from build123d import *

# Parameters (mm, degrees)
SKETCH1_R           = 3.5
BASEHEAD_DEPTH      = 4
SKETCH2_R           = 2
BASEBODY_DEPTH      = 35
HEXAGONSOCKET_DEPTH = 2
TOPFILLET_R         = 0.5
CHAMFER1_SIZE       = 0.2
LPATTERN10_COUNT    = 44
LPATTERN10_PITCH    = 0.4548


with BuildPart() as part:
    # Sketch1 → BaseHead (new body)
    with BuildSketch(Plane(origin=(0, 0, 0), x_dir=(0, 0, -1), z_dir=(1, 0, 0))):
        Circle(SKETCH1_R)
    extrude(amount=BASEHEAD_DEPTH)

    # Sketch2 → BaseBody (add)
    with BuildSketch(Plane(origin=(4, 0, 0), x_dir=(0, 0, -1), z_dir=(1, 0, 0))):
        Circle(SKETCH2_R)
    extrude(amount=BASEBODY_DEPTH)

    # Sketch3 → HexagonSocket (cut)
    with BuildSketch(Plane(origin=(0, 0, 0), x_dir=(0, 0, -1), z_dir=(1, 0, 0))):
        Polygon((1.732050808, 0), (0.866025404, 1.5), (-0.866025404, 1.5), (-1.732050808, 0), (-0.866025404, -1.5), (0.866025404, -1.5), align=None)
    extrude(amount=HEXAGONSOCKET_DEPTH, mode=Mode.SUBTRACT)

    # Sketch4 → Cut-Revolve1 (revolve, cut)
    with BuildSketch(Plane(origin=(-4.19613823, 0.75, 0), x_dir=(-1, 0, 0), z_dir=(0, 0, 1)), mode=Mode.PRIVATE) as cut_revolve1_sk:
        Polygon((-6.19613823, 2.25), (-7.062163633, 0.75), (-6.19613823, 0.75), align=None)
    revolve(cut_revolve1_sk.sketch.rotate(Axis((0.838992387, 0, 0), (-1, 0, 0)), 90), axis=Axis((0.838992387, 0, 0), (-1, 0, 0)), mode=Mode.SUBTRACT)

    # TopFillet
    topfillet_edges = [part.edges().sort_by_distance(p)[0] for p in [
        (0, 0, 3.5),
    ]]
    fillet(topfillet_edges, radius=TOPFILLET_R)

    # Chamfer1
    chamfer1_edges = [part.edges().sort_by_distance(p)[0] for p in [
        (39, 0, 2),
    ]]
    chamfer(chamfer1_edges, length=CHAMFER1_SIZE)

    # Sketch5 → Cut-Revolve10 (revolve, cut)
    with BuildSketch(Plane.XY, mode=Mode.PRIVATE) as cut_revolve10_sk:
        Polygon((38.8, 1.671776372), (38.9895, 2), (38.9895, 2.379), (38.6105, 2.379), (38.6105, 2), align=None)
    cut_revolve10 = revolve(cut_revolve10_sk.sketch.rotate(Axis((0, 0, 0), (1, 0, 0)), 90), axis=Axis((0, 0, 0), (1, 0, 0)), mode=Mode.SUBTRACT)

    # LPattern10: Cut-Revolve10 ×44
    with Locations(*[(-i * LPATTERN10_PITCH, 0, 0) for i in range(1, LPATTERN10_COUNT)]):
        add(cut_revolve10, mode=Mode.SUBTRACT)


solid = part.part
Design review of the part built by this model. Coordinates are the model's own, in mm. Give positions to 0.01 mm unless a question says otherwise; leave off trailing zeros. Loops run counter-clockwise (first coordinate to the right, second up) from the corner with the lowest first, then second, coordinate; pieces in that order, holes last. Notation, with made-up numbers: (-12, 0.25) - (19, 0.25) arc R11 cw to (19, 8.25) - close; hole circle Ø3 at (71, 28). An arc over 180 degrees is marked (long way). Use CSV: the item, a comma, the result in double quotes. Start each with the question number.
1. Draft analysis for pull direction Y (two halves, no side actions). For faces 1 (the flat face through (0.986, -0.74, 1.305)), 2 (the flat face through (0, -1.3, -1.3)), state which applies: released by +Y, released by -Y, zero draft, split by the parting line, or undercut.
2. Add section A-A (x = 14). State the section outline as (y, z) points, plus the area to 3 significant figures.
3. Insertion check: P1, Ø1.5, axis at x = 7.5, z = 1.5, coming from the +Y side; P2, Ø0.6, axis at y = 1, z = -1, coming from the -X side; P3, Ø0.6, axis at y = -1, z = -0.5, coming from the -X side; P4, Ø3, axis at x = 10.5, z = 0, coming from the -Y side. Each pin has a flat end and moves straight along its axis. Give the tip position at first contact, or say it passes through.
4. Wall thickness on L1, parallel to X at y = 2.75, z = -0.5; L2, parallel to Y at x = 21, z = 0; L3, parallel to Z at x = 3.5, y = -1.75: over which ranges is each line inside the solid? List them lowest first.
Results found:
1,face 1,"undercut"
1,face 2,"zero draft"
2,outline,"circle Ø4 at (0, 0)"
2,area,"12.6 mm²"
3,P1,"stops at y = 1.85"
3,P2,"stops at x = 0"
3,P3,"stops at x = 2.05"
3,P4,"stops at y = -2"
4,L1,"x = 0 to 4"
4,L2,"y = -1.78 to 1.78"
4,L3,"z = -3.03 to 3.03"
